from build123d import *

# Parameters (mm, degrees)
CUT_EXTRUDE1_DEPTH = 2.032
SKETCH3_R          = 2.413
EXTRUDE1_DEPTH     = 12.7


with BuildPart() as part:
    # Sketch1 → Revolve1 (revolve)
    with BuildSketch(Plane.XY, mode=Mode.PRIVATE) as revolve1_sk:
        with BuildLine():
            Line((4.5847, 0), (4.5847, 0.635))
            ThreePointArc((4.5847, 0.635), (3.714445355, 1.761301001), (2.54, 2.5654))
            Line((2.54, 2.5654), (0, 2.5654))
            Line((0, 2.5654), (0, 0))
            Line((0, 0), (4.5847, 0))
        make_face()
    revolve(revolve1_sk.sketch.rotate(Axis((0, 0, 0), (0, 1, 0)), 90), axis=Axis((0, 0, 0), (0, 1, 0)))

    # Sketch2 → Cut-Extrude1 (cut)
    with BuildSketch(Plane(origin=(0, 2.5654, 0), x_dir=(-1, 0, 0), z_dir=(0, 1, 0))):
        Polygon((0, 1.833087105), (-1.5875, 0.916543552), (-1.5875, -0.916543552), (0, -1.833087105), (1.5875, -0.916543552), (1.5875, 0.916543552), align=None)
    extrude(amount=-CUT_EXTRUDE1_DEPTH, mode=Mode.SUBTRACT)

    # Sketch3 → Extrude1 (add)
    with BuildSketch(Plane.XZ):
        with Locations(Location((0, 0, 0), (0, 0, 270))):
            Circle(SKETCH3_R)
    extrude(amount=EXTRUDE1_DEPTH)


solid = part.part
The listing builds one solid part. Answer for the finished solid, in the listing's coordinates (mm). A direction names the side the tool comes from. Give positions to 0.01 mm unless a question says otherwise; leave off trailing zeros. Write each loop counter-clockwise with the first axis right and the second up, starting at its lowest first coordinate (ties: lowest second). Pieces come first, ordered by that corner, then holes. Notation, with made-up numbers: (31.25, 55.25) -> (86.25, 55.25) arc R10 ccw to (86.25, 64.25) -> close; hole circle Ø11 at (-5, 49.25). An arc over 180 degrees is marked (long way). One line per question, with ' | ' between items. Start each with the question number.
1. Find the intervals of material crossed by probe 1 along Y at (x, z) = (-1.5, 0.25); probe 2 along Z at (x, y) = (-0.5, 1); probe 3 along Y at (x, z) = (0.5, -4), in increasing order.
2. For a pull along X with two mould halves and no side action, classify faces 1 (the flat face through (-1.588, 2, 0)), 2 (the flat face through (2, 2.565, 0)), 3 (the cylindrical face through (-1.468, -6.261, 1.915)) as pulls with the +X half, pulls with the -X half, needs draft (parallel to the pull), parting line crosses it, or undercut.
3. Section A-A (y = -6.5) is taken. Determine the outline of the cut face in (x, z).
4. Given pin 1 Ø1 at (x, y) = (-1, -4) entering from -Z; pin 2 Ø2 at (y, z) = (-1.5, -1) entering from -X; pin 3 Ø0.5 at (y, z) = (1, 0) entering from -X, each flat-ended and moving along its own axis, determine where each tip first touches the part or whether it passes through.
5. For faces 4 (the cylindrical face through (4.476, 0.322, 0.994)), 5 (the flat face through (2, 0, 2)), 6 (the flat face through (0, 0.533, 0)), determine the directions among +Z, -Z, +X, -X, +Y, -Y from which every point of the face is accessible in a straight line to the end or side of a thin tool.
Response values:
1) probe 1: -12.7 to 0.53 | probe 2: -4.33 to -1.54, 1.54 to 4.33 | probe 3: 0 to 1.43
2) face 1: undercut | face 2: needs draft | face 3: parting line crosses it
3) outline: circle Ø4.83 at (0, 0)
4) pin 1: z = -2.36 | pin 2: x = -2.41 | pin 3: x = -4.52
5) face 4: +Y, -Y | face 5: -Y | face 6: +Y
